Autodesk Inventor part; units mm, degrees
ref_plane "Płaszczyzna konstrukcyjna1" through (0, 0, 24) normal (0, 0, 1) x (1, 0, 0)
ref_plane "YZ Plane" through (0, 0, 0) normal (1, 0, 0) x (0, 1, 0)
ref_plane "XZ Plane" through (0, 0, 0) normal (0, 1, 0) x (-1, 0, 0)
sketch "Szkic1" plane through (0, 0, 0) normal (0, 0, 1) x (1, 0, 0)
  line L0 (-30, -30) -> (30, -30)
  line L1 (30, -30) -> (30, 30)
  line L2 (30, 30) -> (-30, 30)
  line L3 (-30, 30) -> (-30, -30)
  line L4 (-30, -30) -> (30, 30) construction
  line L5 (30, -30) -> (-30, 30) construction
  point P0 (0, 0)
  dimension "d0" = 60
  dimension "d1" = 60
extrude "Wyciągnięcie proste1" add sketch "Szkic1" along normal blind 100
sketch "Szkic2" plane through (0, 0, 100) normal (0, 0, 1) x (1, 0, 0)
  circle A0 centre (0, 0) radius 19.05
  dimension "d4" = 38.1
extrude "Wyciągnięcie proste2" add sketch "Szkic2" along normal blind 1.6
sketch "Szkic3" plane through (0, 0, 100) normal (0, 0, 1) x (1, 0, 0)
  line L0 (0, 0) -> (0, 23.57)
  line L1 (30, -30) -> (30, 30)
  line L2 (-30, 30) -> (-30, -30)
  line L3 (0, 0) -> (0, -23.57)
  line L4 (0, -23.57) -> (23.57, -23.57)
  line L5 (0, -23.57) -> (-23.57, -23.57)
  line L6 (0, 23.57) -> (-23.57, 23.57)
  line L7 (0, 23.57) -> (23.57, 23.57)
  circle A0 centre (23.57, 23.57) radius 2.5
  circle A1 centre (-23.57, 23.57) radius 2.5
  circle A2 centre (-23.57, -23.57) radius 2.5
  circle A3 centre (23.57, -23.57) radius 2.5
  dimension "d13" = 47.14
  dimension "d14" = 47.14
  dimension "d15" = 47.14
  dimension "d16" = 5
  dimension "d17" = 5
  dimension "d18" = 5
  dimension "d19" = 5
extrude "Wyciągnięcie proste3" cut sketch "Szkic3" against normal up to next
sketch "Szkic4" plane through (0, 0, 0) normal (0, 0, -1) x (-1, 0, 0)
  circle A0 centre (23.57, -23.57) radius 2.5
  circle A1 centre (-23.57, 23.57) radius 2.5
  circle A2 centre (23.57, 23.57) radius 2.5
  circle A3 centre (-23.57, -23.57) radius 2.5
  line L0 (30, -30) -> (-30, -30)
  line L1 (30, 30) -> (30, -30)
  line L2 (-30, 30) -> (30, 30)
  line L3 (-30, -30) -> (-30, 30)
  line L4 (-30, -30) -> (-30, 30)
  line L5 (-17, -17) -> (-17, -30)
  line L6 (17, -17) -> (17, -30)
  line L7 (30, 30) -> (30, -30)
  line L8 (-17, -17) -> (-30, -17)
  line L9 (17, 17) -> (30, 17)
  line L10 (-17, 17) -> (-17, 30)
  line L11 (-17, 17) -> (-30, 17)
  line L12 (17, 17) -> (17, 30)
  line L13 (17, -17) -> (30, -17)
  point P0 (0, 0)
extrude "Wyciągnięcie proste4" cut sketch "Szkic4" against normal blind 96 contours L0 L6 L13 L1 | L0 L3 L8 L5 | L9 L12 L2 L1 | L3 L2 L10 L11
sketch "Szkic5" plane through (0, 0, 101.6) normal (0, 0, 1) x (1, 0, 0)
  circle A0 centre (0, 0) radius 3.75
  dimension "d25" = 7.5
extrude "Wyciągnięcie proste5" add sketch "Szkic5" along normal blind 22.5
sketch "Szkic6" plane through (-30, 30, 100) normal (0, 1, 0) x (1, 0, 0)
  line L0 (13, 100) -> (13, 4)
  line L1 (13, 4) -> (0, 4)
  line L2 (0, 4) -> (0, 0)
  line L3 (60, 0) -> (0, 0)
  line L4 (60, 4) -> (60, 0)
  line L5 (60, 4) -> (47, 4)
  line L6 (47, 4) -> (47, 100)
  line L7 (47, 100) -> (13, 100)
  line L8 (13, 4) -> (47, 4)
  line L9 (13, 100) -> (13, 4)
  line L10 (13, 100) -> (13, 96)
  line L11 (13, 96) -> (47, 96)
  point P0 (30, 100)
  dimension "d28" = 4
extrude "Wyciągnięcie proste6" cut sketch "Szkic6" against normal blind 1 contours L11 L6 L8 L0
sketch "Szkic7" plane through (-30, -30, 100) normal (-1, 0, 0) x (0, 0, 1)
  line L0 (-4, 47) -> (-100, 47)
  line L1 (-100, 47) -> (-100, 13)
  line L2 (-100, 13) -> (-4, 13)
  line L3 (-4, 13) -> (-4, 0)
  line L4 (-4, 0) -> (0, 0)
  line L5 (0, 60) -> (0, 0)
  line L6 (-4, 60) -> (0, 60)
  line L7 (-4, 60) -> (-4, 47)
  line L8 (-100, 47) -> (-4, 47)
  line L9 (-100, 13) -> (-4, 13)
  line L10 (-4, 47) -> (-4, 13)
  line L11 (-100, 47) -> (-100, 13)
  line L12 (-96, 13) -> (-96, 47)
  point P0 (-100, 30)
sketch "Szkic8" plane through (-30, -30, 100) normal (0, -1, 0) x (1, 0, 0)
  line L0 (13, -4) -> (13, -100)
  line L1 (13, -100) -> (47, -100)
  line L2 (47, -100) -> (47, -4)
  line L3 (47, -4) -> (60, -4)
  line L4 (60, -4) -> (60, 0)
  line L5 (0, 0) -> (60, 0)
  line L6 (0, -4) -> (0, 0)
  line L7 (0, -4) -> (13, -4)
  line L8 (47, -4) -> (13, -4)
  line L9 (13, -4) -> (47, -4)
  line L10 (47, -100) -> (47, -96)
  line L11 (47, -100) -> (47, -4)
  line L12 (47, -96) -> (13, -96)
  point P0 (30, -100)
  dimension "d34" = 4
sketch "Szkic9" plane through (30, -30, 100) normal (1, 0, 0) x (0, 0, -1)
  line L0 (4, 13) -> (100, 13)
  line L1 (100, 13) -> (100, 47)
  line L2 (100, 47) -> (4, 47)
  line L3 (4, 47) -> (4, 60)
  line L4 (4, 60) -> (0, 60)
  line L5 (0, 0) -> (0, 60)
  line L6 (4, 0) -> (0, 0)
  line L7 (4, 0) -> (4, 13)
  line L8 (4, 47) -> (4, 13)
  line L9 (4, 13) -> (4, 47)
  line L10 (100, 47) -> (100, 60)
  line L11 (100, 47) -> (96, 47)
  line L12 (100, 47) -> (4, 47)
  line L13 (96, 47) -> (96, 13)
  line L14 (100, 13) -> (4, 13)
  point P0 (100, 30)
  dimension "d37" = 4
extrude "Wyciągnięcie proste10" cut sketch "Szkic8" against normal blind 1 contours L8 L2 L12 L0
extrude "Wyciągnięcie proste11" cut sketch "Szkic7" against normal blind 1 contours L10 L2 L12 L0
extrude "Wyciągnięcie proste12" cut sketch "Szkic9" against normal blind 1 contours L8 L2 L13 L0
sketch "Szkic10" plane through (-30, 17, 0) normal (0, 1, 0) x (1, 0, 0)
  line L0 (1, -4) -> (1, -96)
  line L1 (1, -96) -> (13, -96)
  line L2 (13, -4) -> (13, -96)
  line L3 (1, -4) -> (1, -96)
  line L4 (1, -4) -> (13, -4)
  point P0 (30, 0)
extrude "Wyciągnięcie proste13" cut sketch "Szkic10" against normal blind 1
sketch "Szkic11" plane through (-17, 17, 0) normal (-1, 0, 0) x (0, 0, 1)
  line L0 (4, 0) -> (4, -1)
  line L1 (4, -1) -> (96, -1)
  line L2 (96, -1) -> (96, 12)
  line L3 (96, 12) -> (4, 12)
  line L4 (96, 12) -> (4, 12)
  line L5 (4, 12) -> (4, 0)
  point P0 (0, -17)
extrude "Wyciągnięcie proste14" cut sketch "Szkic11" against normal blind 1
sketch "Szkic12" plane through (17, 17, 0) normal (0, 1, 0) x (1, 0, 0)
  line L0 (12, -96) -> (12, -4)
  line L1 (0, -4) -> (0, -96)
  line L2 (0, -96) -> (12, -96)
  line L3 (12, -4) -> (0, -4)
  point P0 (-17, 0)
extrude "Wyciągnięcie proste15" cut sketch "Szkic12" against normal blind 1
sketch "Szkic13" plane through (17, 17, 0) normal (1, 0, 0) x (0, 0, -1)
  line L0 (-4, 12) -> (-96, 12)
  line L1 (-96, 12) -> (-96, -1)
  line L2 (-96, -1) -> (-4, -1)
  line L3 (-4, 0) -> (-4, -1)
  line L4 (-4, -1) -> (-4, 12)
  line L5 (-4, 0) -> (-4, 12)
  point P0 (0, -17)
extrude "Wyciągnięcie proste16" cut sketch "Szkic13" against normal blind 1
sketch "Szkic14" plane through (17, -17, 0) normal (0, -1, 0) x (1, 0, 0)
  line L0 (12, 4) -> (12, 96)
  line L1 (12, 96) -> (0, 96)
  line L2 (0, 4) -> (0, 96)
  line L3 (0, 4) -> (12, 4)
  line L4 (-1, 4) -> (-1, 96)
  point P0 (-17, 0)
extrude "Wyciągnięcie proste17" cut sketch "Szkic14" against normal blind 1
sketch "Szkic15" plane through (17, -30, 0) normal (1, 0, 0) x (0, 0, -1)
  line L0 (-96, 1) -> (-4, 1)
  line L1 (-4, 13) -> (-4, 14)
  line L2 (-4, 14) -> (-96, 14)
  line L3 (-96, 14) -> (-96, 1)
  line L4 (-4, 1) -> (-96, 1)
  line L5 (-4, 1) -> (-4, 13)
  point P0 (0, 30)
extrude "Wyciągnięcie proste18" cut sketch "Szkic15" against normal blind 1
sketch "Szkic16" plane through (-30, -17, 0) normal (0, -1, 0) x (1, 0, 0)
  line L0 (1, 96) -> (1, 4)
  line L1 (13, 4) -> (13, 96)
  line L2 (13, 96) -> (1, 96)
  line L3 (1, 4) -> (14, 4)
  line L4 (13, 4) -> (1, 4)
  point P0 (30, 0)
extrude "Wyciągnięcie proste19" cut sketch "Szkic16" against normal blind 1
sketch "Szkic17" plane through (-17, -30, 0) normal (-1, 0, 0) x (0, 0, 1)
  line L0 (4, 1) -> (96, 1)
  line L1 (96, 1) -> (96, 14)
  line L2 (96, 14) -> (4, 14)
  line L3 (4, 13) -> (4, 14)
  line L4 (4, 14) -> (4, 1)
  line L5 (4, 13) -> (4, 1)
  point P0 (0, 30)
extrude "Wyciągnięcie proste20" cut sketch "Szkic17" against normal blind 1
fillet "Zaokrąglenie1" radius 5 28 edges at (-30, 30, 98) (30, 30, 98) (30, -30, 98) (-30, -30, 98) (-16, -16, 50) (-29, -16, 50) (-16, -29, 50) (16, -29, 50) (16, -16, 50) (29, -16, 50) (29, 16, 50) (16, 16, 50) (16, 29, 50) (-16, 29, 50) (-16, 16, 50) (-29, 16, 50) (-30, 17, 2) (-17, 17, 2) (-17, 30, 2) (17, 30, 2) (17, 17, 2) (30, 17, 2) (30, -17, 2) (17, -17, 2) (17, -30, 2) (-17, -30, 2) (-17, -17, 2) (-30, -17, 2)
ref_plane "Płaszczyzna konstrukcyjna1" through (0, 0, 24) normal (0, 0, 1) x (1, 0, 0)
sketch "Szkic19" plane through (0, 0, 24) normal (0, 0, 1) x (1, 0, 0)
  arc A0 (-30, -12) -> (-25, -17) centre (-25, -12) ccw
  line L0 (-30, 12) -> (-30, -12)
  arc A1 (-25, 17) -> (-30, 12) centre (-25, 12) ccw
  line L1 (-25, 17) -> (-22, 17)
  arc A2 (-22, 17) -> (-17, 22) centre (-22, 22) ccw
  line L2 (-17, 22) -> (-17, 25)
  arc A3 (-12, 30) -> (-17, 25) centre (-12, 25) ccw
  line L3 (12, 30) -> (-12, 30)
  arc A4 (17, 25) -> (12, 30) centre (12, 25) ccw
  line L4 (17, 25) -> (17, 22)
  arc A5 (17, 22) -> (22, 17) centre (22, 22) ccw
  line L5 (22, 17) -> (25, 17)
  arc A6 (30, 12) -> (25, 17) centre (25, 12) ccw
  line L6 (30, -12) -> (30, 12)
  arc A7 (25, -17) -> (30, -12) centre (25, -12) ccw
  line L7 (25, -17) -> (22, -17)
  arc A8 (22, -17) -> (17, -22) centre (22, -22) ccw
  line L8 (17, -22) -> (17, -25)
  arc A9 (12, -30) -> (17, -25) centre (12, -25) ccw
  line L9 (-12, -30) -> (12, -30)
  arc A10 (-17, -25) -> (-12, -30) centre (-12, -25) ccw
  line L10 (-17, -25) -> (-17, -22)
  arc A11 (-17, -22) -> (-22, -17) centre (-22, -22) ccw
  line L11 (-22, -17) -> (-25, -17)
  point P0 (0, 0)
extrude "Wyciągnięcie proste21" add sketch "Szkic19" along normal blind 4
split "Podział1" plane through (0, 0, 24) removes the side toward (0, 0, -1)
properties part number "Silnik krokowy SM 60 100-4004AF - 4Nm"
Model file for the job. Use its own axes, mm. A direction names the side the tool comes from. Give positions to 0.01 mm unless a question says otherwise; leave off trailing zeros. Loops run counter-clockwise (first coordinate to the right, second up) from the corner with the lowest first, then second, coordinate; pieces in that order, holes last. Notation, with made-up numbers: (-18, -38) -> (19, -38) arc R7 ccw to (19, -29) -> close; hole circle Ø4 at (46, 76). An arc over 180 degrees is marked (long way). Use a Markdown table: item, result. Add a question column.
(1) Slice it at C-C on z = 60.5. List the corners of the cut face in (x, y), and give its area (3 significant figures).
(2) Mould opens along Z. For faces 1 (the cylindrical face through (-27, -15, 62)), 2 (the flat face through (0, 0, 124.1)), 3 (the flat face through (-17, 23, 26)) say: +Z half, -Z half, draft (parallel to the pull), parting line (faces both ways), or undercut.
(3) Drop flat-ended pins along their axis: pin 1 Ø1.5 at (x, z) = (-24, 25) entering from -Y; pin 2 Ø17.5 at (y, z) = (-3, 78.5) entering from -X; pin 3 Ø5 at (y, z) = (2.5, 103.5) entering from -X. Give the stop position or say it passes through.
(4) Tool access for faces 4 (the flat face through (24, -17, 26)), 5 (the cylindrical face through (-28, -16, 26)), 6 (the cylindrical face through (-3.746, -0.165, 112.692)), 7 (the flat face through (17, 24, 26)), 8 (the flat face through (-24, 17, 26)): list every direction of +Z, -Z, +X, -X, +Y, -Y with a clear straight run to the whole face (end or side of a thin tool).
(5) Slice it at A-A on z = 98.5. List the corners of the cut face in (x, y).
(6) Slice it at B-B on y = 0. List the corners of the cut face in (x, z).
(7) Wall check: line 1 along Y through (x, z) = (-23.57, 97.05); line 2 along Y through (x, z) = (-23, 97); line 3 along X through (y, z) = (8, 35.5). Give the ranges that are in metal, low to high.
(8) Slice it at D-D on x = 7.5. List the corners of the cut face in (y, z).
Filled sheet:
| question | item | result |
|---|---|---|
| 1 | outline | (-29, -11) arc R5 ccw to (-24, -16) -> (-21, -16) arc R5 cw to (-16, -21) -> (-16, -24) arc R5 ccw to (-11, -29) -> (11, -29) arc R5 ccw to (16, -24) -> (16, -21) arc R5 cw to (21, -16) -> (24, -16) arc R5 ccw to (29, -11) -> (29, 11) arc R5 ccw to (24, 16) -> (21, 16) arc R5 cw to (16, 21) -> (16, 24) arc R5 ccw to (11, 29) -> (-11, 29) arc R5 ccw to (-16, 24) -> (-16, 21) arc R5 cw to (-21, 16) -> (-24, 16) arc R5 ccw to (-29, 11) -> close |
| 1 | area | 2,670 mm2 |
| 2 | face 1 | undercut |
| 2 | face 2 | +Z half |
| 2 | face 3 | draft |
| 3 | pin 1 | y = -17 |
| 3 | pin 2 | x = -29 |
| 3 | pin 3 | x = -19.03 |
| 4 | face 4 | -Z, +X, -Y |
| 4 | face 5 | -Z, -X, -Y |
| 4 | face 6 | +Z |
| 4 | face 7 | -Z, +X, +Y |
| 4 | face 8 | -Z, -X, +Y |
| 5 | outline | (-30, -25) arc R5 ccw to (-25, -30) -> (25, -30) arc R5 ccw to (30, -25) -> (30, 25) arc R5 ccw to (25, 30) -> (-25, 30) arc R5 ccw to (-30, 25) -> close; hole circle Ø5 at (-23.57, -23.57); hole circle Ø5 at (-23.57, 23.57); hole circle Ø5 at (23.57, -23.57); hole circle Ø5 at (23.57, 23.57) |
| 6 | outline | (-30, 24) -> (30, 24) -> (30, 28) -> (29, 28) -> (29, 96) -> (30, 96) -> (30, 100) -> (19.05, 100) -> (19.05, 101.6) -> (3.75, 101.6) -> (3.75, 124.1) -> (-3.75, 124.1) -> (-3.75, 101.6) -> (-19.05, 101.6) -> (-19.05, 100) -> (-30, 100) -> (-30, 96) -> (-29, 96) -> (-29, 28) -> (-30, 28) -> close |
| 7 | line 1 | -30 to -26.07, -21.07 to 21.07, 26.07 to 30 |
| 7 | line 2 | -30 to -26, -21.14 to 21.14, 26 to 30 |
| 7 | line 3 | -29 to 29 |
| 8 | outline | (-30, 24) -> (30, 24) -> (30, 28) -> (29, 28) -> (29, 96) -> (30, 96) -> (30, 100) -> (17.51, 100) -> (17.51, 101.6) -> (-17.51, 101.6) -> (-17.51, 100) -> (-30, 100) -> (-30, 96) -> (-29, 96) -> (-29, 28) -> (-30, 28) -> close |
